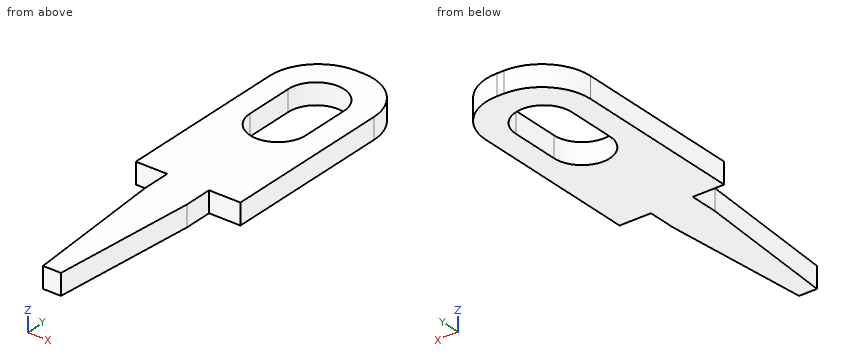
```python
from build123d import *

# Parameters (mm, degrees)
ESTRUSIONE_ESTRUSIONE1_DEPTH = 0.6


with BuildPart() as part:
    # Schizzo1 → Estrusione-Estrusione1 (new body)
    with BuildSketch(Plane.XY):
        with BuildLine():
            Line((-1.5, 0), (-0.6, 0))
            Line((-0.6, 0), (-0.6, -0.808174013))
            Line((-0.6, -0.808174013), (-0.257137319, -5))
            Line((-0.257137319, -5), (0.257137319, -5))
            Line((0.257137319, -5), (0.6, -0.808174013))
            Line((0.6, -0.808174013), (0.6, 0))
            Line((0.6, 0), (1.5, 0))
            Line((1.5, 0), (1.5, 4.9))
            ThreePointArc((1.5, 4.9), (1.089949494, 5.889949494), (0.1, 6.3))
            Line((0.1, 6.3), (-0.1, 6.3))
            ThreePointArc((-0.1, 6.3), (-1.089949494, 5.889949494), (-1.5, 4.9))
            Line((-1.5, 4.9), (-1.5, 0))
        make_face()
        with BuildLine():
            Line((0.8, 4.7), (0.8, 3.3))
            ThreePointArc((0.8, 3.3), (0, 2.5), (-0.8, 3.3))
            Line((-0.8, 3.3), (-0.8, 4.7))
            ThreePointArc((-0.8, 4.7), (0, 5.5), (0.8, 4.7))
        make_face(mode=Mode.SUBTRACT)
    extrude(amount=ESTRUSIONE_ESTRUSIONE1_DEPTH)


solid = part.part
```
Geometry check sheet. Reference: the model listing, model coordinates, mm. Round coordinates to 2 decimals unless told otherwise and drop trailing zeros. Order: outer loops, then holes, each group sorted by start corner. A loop starts at its lowest first (then second) coordinate and runs counter-clockwise, first axis right, second up. Notation, with made-up numbers: (14, 65.5) -> (53, 65.5) arc R33 ccw to (53, 95.5) -> close; hole circle Ø6 at (32, 65.5). An arc over 180 degrees is marked (long way). Return JSON: item names as keys, results as strings. Group by question number.
Q1. Section check A-A, the plane x = 0. Record the boundary of the cut face in (y, z).
Q2. Section check C-C, the plane z = 0.15. Record the boundary of the cut face in (x, y), plus the area to 3 significant figures.
Q3. Section check D-D, the plane x = -1.25. Record the boundary of the cut face in (y, z).
Q4. Material ranges on probe 1 along X at (y, z) = (3.25, 0.5); probe 2 along X at (y, z) = (5.25, 0.15); probe 3 along X at (y, z) = (-3.5, 0.1), recorded low to high. Write a range as from..to.
Q5. Section check B-B, the plane y = 4. Record the boundary of the cut face in (x, z), plus the area to 3 significant figures.
Numbers:
{
 "1": {"outline": "(-5, 0) -> (2.5, 0) -> (2.5, 0.6) -> (-5, 0.6) -> close; (5.5, 0) -> (6.3, 0) -> (6.3, 0.6) -> (5.5, 0.6) -> close"},
 "2": {"outline": "(-1.5, 0) -> (-0.6, 0) -> (-0.6, -0.81) -> (-0.26, -5) -> (0.26, -5) -> (0.6, -0.81) -> (0.6, 0) -> (1.5, 0) -> (1.5, 4.9) arc R1.4 ccw to (0.1, 6.3) -> (-0.1, 6.3) arc R1.4 ccw to (-1.5, 4.9) -> close; hole (-0.8, 3.3) arc R0.8 ccw to (0.8, 3.3) -> (0.8, 4.7) arc R0.8 ccw to (-0.8, 4.7) -> close", "area": "18.4 mm^2"},
 "3": {"outline": "(0, 0) -> (5.7, 0) -> (5.7, 0.6) -> (0, 0.6) -> close"},
 "4": {"probe 1": "-1.5..-0.8, 0.8..1.5", "probe 2": "-1.46..-0.58, 0.58..1.46", "probe 3": "-0.38..0.38"},
 "5": {"outline": "(-1.5, 0) -> (-0.8, 0) -> (-0.8, 0.6) -> (-1.5, 0.6) -> close; (0.8, 0) -> (1.5, 0) -> (1.5, 0.6) -> (0.8, 0.6) -> close", "area": "0.840 mm^2"}
}
